from build123d import *

# Parameters (mm, degrees)
SKETCH1_W               = 50
SKETCH1_H               = 50
BOSS_EXTRUDE1_DEPTH     = 3
CUT_EXTRUDE1_DEPTH      = 71.774289117
CUT_EXTRUDE1_DEPTH_BACK = 71.774289117
SKETCH2_R               = 11
CUT_EXTRUDE2_DEPTH      = 71.774289117
CUT_EXTRUDE2_DEPTH_BACK = 71.774289117
SKETCH3_R               = 1.78
FILLET1_R               = 1.5
SKETCH4_W               = 15.5
SKETCH4_H               = 15.5
SKETCH4_R               = 2.35
BOSS_EXTRUDE3_DEPTH     = 10
BOSS_EXTRUDE4_START     = 4
SKETCH6_W               = 15.5
SKETCH6_H               = 15.5
SKETCH6_R               = 2.35
BOSS_EXTRUDE4_DEPTH     = 4
FILLET3_SIZE            = 3.3


with BuildPart() as part:
    # Sketch1 → Boss-Extrude1 (new body)
    with BuildSketch(Plane(origin=(0, 0, 0), x_dir=(1, 0, 0), z_dir=(0, 1, 0))):
        with Locations((25, -25)):
            Rectangle(SKETCH1_W, SKETCH1_H)
    extrude(amount=BOSS_EXTRUDE1_DEPTH)

    # Sketch2 → Cut-Extrude1 (cut, two sides: drawn at the far end of the back side and taken through both)
    with BuildSketch(Plane(origin=(0, 3, 0), x_dir=(1, 0, 0), z_dir=(0, 1, 0)).offset(-CUT_EXTRUDE1_DEPTH_BACK)):
        with Locations(Location((25, -25, 0), (0, 0, 270))):
            Circle(SKETCH2_R)
    extrude(amount=CUT_EXTRUDE1_DEPTH + CUT_EXTRUDE1_DEPTH_BACK, mode=Mode.SUBTRACT)

    # Sketch3 → Cut-Extrude2 (cut, two sides: drawn at the far end of the back side and taken through both)
    with BuildSketch(Plane(origin=(0, 3, 0), x_dir=(1, 0, 0), z_dir=(0, 1, 0)).offset(-CUT_EXTRUDE2_DEPTH_BACK)):
        with Locations(Location((9.47, -11.25, 0), (0, 0, 270))):
            Circle(SKETCH3_R)
        with Locations(Location((40.53, -11.25, 0), (0, 0, 270))):
            Circle(SKETCH3_R)
        with Locations(Location((40.53, -38.75, 0), (0, 0, 270))):
            Circle(SKETCH3_R)
        with Locations(Location((9.47, -38.75, 0), (0, 0, 270))):
            Circle(SKETCH3_R)
    extrude(amount=CUT_EXTRUDE2_DEPTH + CUT_EXTRUDE2_DEPTH_BACK, mode=Mode.SUBTRACT)

    # Fillet1
    fillet1_edges = [part.edges().sort_by_distance(p)[0] for p in [
        (25, 0, 14),
    ]]
    fillet(fillet1_edges, radius=FILLET1_R)

    # Sketch4 → Boss-Extrude3 (add)
    # profile 1 of 2: a face of its own
    with BuildSketch(Plane.XZ):
        with Locations((-7.75, 25)):
            Rectangle(SKETCH4_W, SKETCH4_H)
        with Locations(Location((-7.75, 25, 0), (0, 0, 270))):
            Circle(SKETCH4_R, mode=Mode.SUBTRACT)
    # profile 2 of 2: a face of its own
    with BuildSketch(Plane.XZ):
        with Locations((57.75, 25)):
            Rectangle(SKETCH4_W, SKETCH4_H)
        with Locations(Location((57.75, 25, 0), (0, 0, 270))):
            Circle(SKETCH4_R, mode=Mode.SUBTRACT)
    extrude(amount=-BOSS_EXTRUDE3_DEPTH)

    # Sketch6 → Boss-Extrude4 (add)
    # profile 1 of 2: a face of its own
    with BuildSketch(Plane.XZ.offset(BOSS_EXTRUDE4_START)):
        with Locations((-7.75, 25)):
            Rectangle(SKETCH6_W, SKETCH6_H)
        with Locations(Location((-7.75, 25, 0), (0, 0, 270))):
            Circle(SKETCH6_R, mode=Mode.SUBTRACT)
    # profile 2 of 2: a face of its own
    with BuildSketch(Plane.XZ.offset(BOSS_EXTRUDE4_START)):
        with Locations((57.75, 25)):
            Rectangle(SKETCH6_W, SKETCH6_H)
        with Locations(Location((57.75, 25, 0), (0, 0, 270))):
            Circle(SKETCH6_R, mode=Mode.SUBTRACT)
    extrude(amount=-BOSS_EXTRUDE4_DEPTH)

    # Fillet3
    # a fillet whose section is not a circle: 3.3 mm, written as the material it takes off along each edge
    with BuildSketch(Plane(origin=(-7.75, 10, 25), x_dir=(0, 0, -1), z_dir=(-1, 0, 0))) as fillet3_piece_1:
        with BuildLine():
            Bezier((2.35, FILLET3_SIZE), (2.35, 0), (2.35 + FILLET3_SIZE, 0), weights=[1, 0.016667517, 1])
            Line((2.35 + FILLET3_SIZE, 0), (2.35, 0))
            Line((2.35, 0), (2.35, FILLET3_SIZE))
        make_face()
    revolve(axis=Axis((-7.75, 10, 25), (0, -1, 0)), mode=Mode.SUBTRACT)
    with BuildSketch(Plane(origin=(57.75, 10, 25), x_dir=(0, 0, -1), z_dir=(-1, 0, 0))) as fillet3_piece_2:
        with BuildLine():
            Bezier((2.35, FILLET3_SIZE), (2.35, 0), (2.35 + FILLET3_SIZE, 0), weights=[1, 0.016667517, 1])
            Line((2.35 + FILLET3_SIZE, 0), (2.35, 0))
            Line((2.35, 0), (2.35, FILLET3_SIZE))
        make_face()
    revolve(axis=Axis((57.75, 10, 25), (0, -1, 0)), mode=Mode.SUBTRACT)


solid = part.part
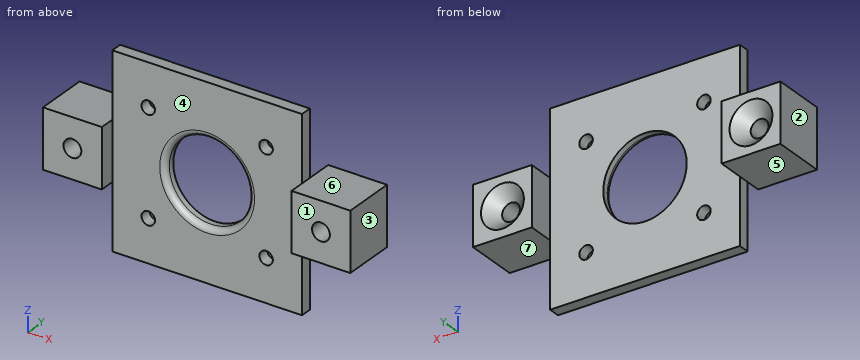
The model under review builds one solid part; all positions refer to its coordinate system, in mm. Face numbers are marked on the shaded views. A direction names the side the tool comes from. Give positions to 0.01 mm unless a question says otherwise; leave off trailing zeros. Order: outer loops, then holes, each group sorted by start corner. A loop starts at its lowest first (then second) coordinate and runs counter-clockwise, first axis right, second up. Notation, with made-up numbers: (24.5, 33.25) -> (45.5, 33.25) arc R12 cw to (45.5, 50.25) -> close; hole circle Ø9 at (59, 41.25). An arc over 180 degrees is marked (long way). Write item = value, one per line. Start each with the question number.
(1) Take a section at D-D (x = 25). Write out the cut boundary in (y, z).
(2) Take a section at B-B (x = 40.53). Write out the cut boundary in (y, z), plus the area to 3 significant figures.
(3) Tool access review of the marked faces 5, 6 and 7: name each direction out of +Z, -Z, +X, -X, +Y, -Y from which nothing blocks a thin tool from reaching the whole face with its end or side.
(4) Take a section at A-A (y = -1.5). Write out the cut boundary in (x, z).
(5) Take a section at C-C (z = 38.75). Write out the cut boundary in (x, y).
(6) For pin 1 Ø6 at (x, z) = (39, 38) entering from +Y; pin 2 Ø8 at (x, z) = (16.5, 33.5) entering from -Y; pin 3 Ø4 at (y, z) = (-0.5, 11) entering from -X; pin 4 Ø3 at (x, z) = (9.47, 38.75) entering from +Y, all flat-tipped, find the tip position at first contact; note any pin that passes through.
(7) Draft analysis for pull direction X (two halves, no side actions). For the marked faces 1, 2, 3 and 4, state which applies: +X half, -X half, draft (parallel to the pull), parting line (faces both ways), or undercut.
(8) For L1, parallel to Z at x = 9.47, y = 1.45; L2, parallel to X at y = 2.05, z = 11.25; L3, parallel to X at y = 1.5, z = 25, list the stretches that pass through material, from the lowest coordinate up. Write a range as from..to.
Returned:
q1.outline = (0, 0) -> (3, 0) -> (3, 14) -> (1.5, 14) arc R1.5 ccw to (0, 12.5) -> close; (0, 37.5) arc R1.5 ccw to (1.5, 36) -> (3, 36) -> (3, 50) -> (0, 50) -> close
q2.outline = (0, 0) -> (3, 0) -> (3, 9.47) -> (0, 9.47) -> close; (0, 13.03) -> (3, 13.03) -> (3, 36.97) -> (0, 36.97) -> close; (0, 40.53) -> (3, 40.53) -> (3, 50) -> (0, 50) -> close
q2.area = 129 mm²
q3.face_5 = -Z, -X, +Y, -Y
q3.face_6 = +Z, +X, +Y, -Y
q3.face_7 = -Z, +X, +Y, -Y
q4.outline = (-15.5, 17.25) -> (0, 17.25) -> (0, 32.75) -> (-15.5, 32.75) -> close; (50, 17.25) -> (65.5, 17.25) -> (65.5, 32.75) -> (50, 32.75) -> close; hole circle Ø4.7 at (-7.75, 25); hole circle Ø4.7 at (57.75, 25)
q5.outline = (0, 0) -> (7.69, 0) -> (7.69, 3) -> (0, 3) -> close; (11.25, 0) -> (38.75, 0) -> (38.75, 3) -> (11.25, 3) -> close; (42.31, 0) -> (50, 0) -> (50, 3) -> (42.31, 3) -> close
q6.pin_1 = 3
q6.pin_2 = 0
q6.pin_3 = 0
q6.pin_4 = through
q7.face_1 = draft
q7.face_2 = -X half
q7.face_3 = +X half
q7.face_4 = undercut
q8.L1 = 0..9.47, 13.03..36.97, 40.53..50
q8.L2 = 0..7.69, 11.25..38.75, 42.31..50
q8.L3 = -15.5..-10.1, -5.4..14, 36..55.4, 60.1..65.5
